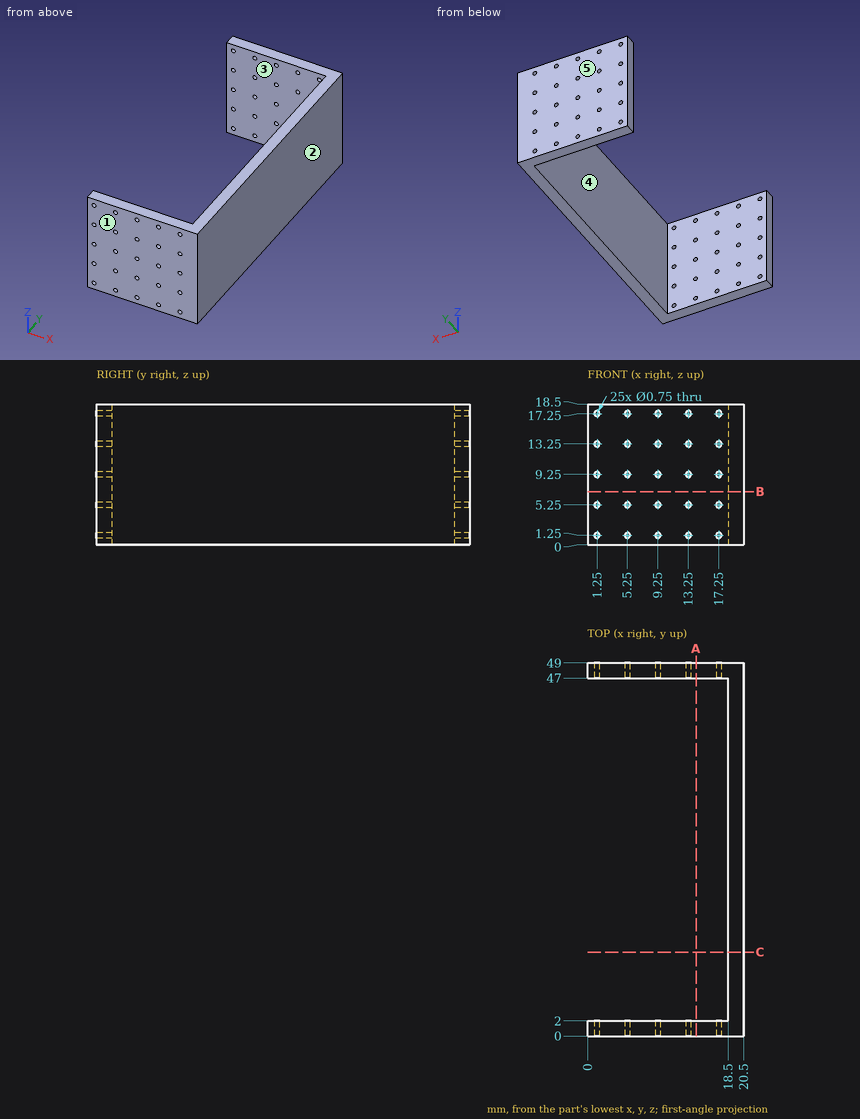
The figure shows three views and two pictorial views of one solid part (mm, origin at its lowest corner). Answer the questions. A direction names the side the tool comes from. Give positions to 0.01 mm unless a question says otherwise; leave off trailing zeros. Loops run counter-clockwise (first coordinate to the right, second up) from the corner with the lowest first, then second, coordinate; pieces in that order, holes last. Notation, with made-up numbers: (71, 7) -> (79, 7) arc R4 ccw to (79, 11) -> close; hole circle Ø11 at (50, -7). An arc over 180 degrees is marked (long way). Use a Markdown table: item, result. Add a question column.
1. Find the intervals of material crossed by probe 1 along Z at (x, y) = (9.25, 47.7) (3 decimals); probe 2 along Y at (x, z) = (14.75, 17.5); probe 3 along X at (y, z) = (32.5, 1.5), in increasing order.
2. Section A-A on x = 14.25 is taken. Determine the outline of the cut face in (y, z), and give its area (3 significant figures).
3. Section C-C on y = 11 is taken. Determine the outline of the cut face in (x, z).
4. For the marked faces 4 and 5, determine the directions among +Z, -Z, +X, -X, +Y, -Y from which every point of the face is accessible in a straight line to the end or side of a thin tool.
5. Section B-B on z = 7 is taken. Determine the outline of the cut face in (x, y).
6. A flat-ended cylindrical pin translates along its axis: pin 1 Ø9 at (y, z) = (35.5, 7) entering from -X. Find the tip coordinate at first contact, or state that the pin passes through.
7. Determine the mould class of the marked faces 1, 2 and 3 for opening direction Y: released by +Y, released by -Y, zero draft, split by the parting line, or undercut.
Results below:
| question | item | result |
|---|---|---|
| 1 | probe 1 | z = 0 to 0.875, 1.625 to 4.875, 5.625 to 8.875, 9.625 to 12.875, 13.625 to 16.875, 17.625 to 18.5 |
| 1 | probe 2 | y = 0 to 2, 47 to 49 |
| 1 | probe 3 | x = 18.5 to 20.5 |
| 2 | outline | (0, 0) -> (2, 0) -> (2, 18.5) -> (0, 18.5) -> close; (47, 0) -> (49, 0) -> (49, 18.5) -> (47, 18.5) -> close |
| 2 | area | 74.0 mm^2 |
| 3 | outline | (18.5, 0) -> (20.5, 0) -> (20.5, 18.5) -> (18.5, 18.5) -> close |
| 4 | face 4 | +Z, -Z, -X |
| 4 | face 5 | +Z, -Z, +X, -X, +Y |
| 5 | outline | (0, 0) -> (20.5, 0) -> (20.5, 49) -> (0, 49) -> (0, 47) -> (18.5, 47) -> (18.5, 2) -> (0, 2) -> close |
| 6 | pin 1 | stops at x = 18.5 |
| 7 | face 1 | released by -Y |
| 7 | face 2 | zero draft |
| 7 | face 3 | undercut |
